Verification items for the finished model (mm, model axes). A direction names the side the tool comes from. Give positions to 0.01 mm unless a question says otherwise; leave off trailing zeros. Loops run counter-clockwise (first coordinate to the right, second up) from the corner with the lowest first, then second, coordinate; pieces in that order, holes last. Notation, with made-up numbers: (56, 85) -> (112, 85) arc R6 ccw to (112, 95) -> close; hole circle Ø11 at (82.25, -28.5). An arc over 180 degrees is marked (long way). Answer in a Markdown table with one row per item. Add a question column.
Q1. Set-up check for faces 1 (the face through (-66.1, 6, 12.7)), 2 (the face through (71, 0, 12.7)), 3 (the face through (0, 0, 25.4)): record each of +Z, -Z, +X, -X, +Y, -Y from which the full face is reachable in a straight line by a thin tool's end or side.
Q2. Section check D-D on y = 23. Enter the section's corners in (x, z).
Q3. Section check B-B on z = 10.5. Enter the section's corners in (x, y).
Q4. Gauge pin test, flat ends, axial feed: P1, Ø4, axis at x = -51.5, z = 6, coming from the -Y side; P2, Ø4, axis at x = 56.5, z = 5.5, coming from the +Y side; P3, Ø23, axis at x = 72, y = -5.5, coming from the +Z side. Record the tip position at first contact, or that the pin passes through.
Q5. Material ranges on probe 1 along Y at (x, z) = (63, 8); probe 2 along Z at (x, y) = (-52, -19); probe 3 along X at (y, z) = (29, 12), recorded low to high.
Q6. Section check C-C on x = 0. Enter the section's corners in (y, z).
Q7. Section check A-A on y = 0. Enter the section's corners in (x, z), and give its area (3 significant figures).
Autodesk Fusion 360 part; units mm, degrees
sketch "Sketch1" plane through (0, 0, 0) normal (0, 0, 1) x (1, 0, 0) in component "u-Bracket"
  line L0 (-63.5, -25.4) -> (63.5, -25.4)
  arc A0 (63.5, -25.4) -> (63.5, 25.4) centre (63.5, 0) ccw
  line L1 (63.5, 25.4) -> (-63.5, 25.4)
  arc A1 (-63.5, 25.4) -> (-63.5, -25.4) centre (-63.5, 0) ccw
  line L2 (-63.5, 0) -> (63.5, 0) construction
  circle A2 centre (63.5, 0) radius 6.35
  circle A3 centre (-63.5, 0) radius 6.35
  dimension "d1" = 127
  dimension "d2" = 12.7
  dimension "d3" = 12.7
  dimension "d4" = 25.4
  dimension "d5" = 63.5
extrude "Extrude2" add sketch "Sketch1" along normal blind 12.7 makes body 1 in component "u-Bracket"
extrude "Extrude1" add sketch "Sketch1" along normal blind 12.7 separate body makes body 2 in component "u-Bracket"
sketch "Sketch2" plane through (0, 0, 0) normal (0, 1, 0) x (1, 0, 0) in component "u-Bracket"
  circle A0 centre (0, 0) radius 44.45
  line L0 (-44.45, 0) -> (44.45, 0)
  dimension "d10" = 88.9
extrude "Extrude3" add sketch "Sketch2" along normal mid plane 63.5 contours A0 L0 picked at (-7.4083, -12.8316) bodies 1 2 in component "u-Bracket"
sketch "Sketch3" plane through (0, -31.75, 0) normal (0, -1, 0) x (1, 0, 0) in component "u-Bracket"
  arc A0 (44.45, 0) -> (-44.45, 0) centre (0, 0) ccw
  line L0 (-44.45, 0) -> (44.45, 0)
  line L1 (-25.4, 0) -> (25.4, 0)
  line L2 (25.4, 0) -> (25.4, 25.4)
  line L3 (25.4, 25.4) -> (-25.4, 25.4)
  line L4 (-25.4, 25.4) -> (-25.4, 0)
  line L5 (-63.5, 0) -> (63.5, 0)
  dimension "d13" = 50.8
  dimension "d14" = 25.4
extrude "Extrude4" cut sketch "Sketch3" against normal through all contours L0 L1 L2 L3 L4 L5 bodies 1 in component "u-Bracket"
sketch "Sketch4" plane through (0, 0, 25.4) normal (0, 0, -1) x (1, 0, 0) in component "u-Bracket"
  line L0 (-25.4, -31.75) -> (25.4, -31.75)
  line L1 (25.4, -31.75) -> (25.4, 31.75)
  line L2 (25.4, 31.75) -> (-25.4, 31.75)
  line L3 (-25.4, 31.75) -> (-25.4, -31.75)
  circle A0 centre (0, 0) radius 3.175
  dimension "d16" = 6.35
extrude "Extrude5" cut sketch "Sketch4" along normal through all contours A0 bodies 1 in component "u-Bracket"
component "u-Bracket" placed x (1, 0, 0) y (0, 1, 0) z (0, 0, 1) at (0, 0, 0)
equation "d5 = d1 / 2"
Taken from the geometry:
| question | item | result |
|---|---|---|
| 1 | face 1 | +Z, -X, +Y, -Y |
| 1 | face 2 | +Z, +X, +Y, -Y |
| 1 | face 3 | -Z, +Y, -Y |
| 2 | outline | (-74.28, 0) -> (-25.4, 0) -> (-25.4, 25.4) -> (25.4, 25.4) -> (25.4, 0) -> (74.28, 0) -> (74.28, 12.7) -> (42.6, 12.7) arc R44.45 ccw to (-42.6, 12.7) -> (-74.28, 12.7) -> close |
| 3 | outline | (-63.5, -25.4) -> (-43.19, -25.4) -> (-43.19, -31.75) -> (-25.4, -31.75) -> (-25.4, 31.75) -> (-43.19, 31.75) -> (-43.19, 25.4) -> (-63.5, 25.4) arc R25.4 ccw to start; (25.4, -31.75) -> (43.19, -31.75) -> (43.19, -25.4) -> (63.5, -25.4) arc R25.4 ccw to (63.5, 25.4) -> (43.19, 25.4) -> (43.19, 31.75) -> (25.4, 31.75) -> close; hole circle Ø12.7 at (-63.5, 0); hole circle Ø12.7 at (63.5, 0) |
| 4 | P1 | stops at y = -25.4 |
| 4 | P2 | stops at y = 25.4 |
| 4 | P3 | stops at z = 12.7 |
| 5 | probe 1 | y = -25.4 to -6.33, 6.33 to 25.4 |
| 5 | probe 2 | z = 0 to 12.7 |
| 5 | probe 3 | x = -42.8 to -25.4, 25.4 to 42.8 |
| 6 | outline | (-31.75, 25.4) -> (31.75, 25.4) -> (31.75, 44.45) -> (-31.75, 44.45) -> close |
| 7 | outline | (-88.9, 0) -> (-69.85, 0) -> (-69.85, 12.7) -> (-88.9, 12.7) -> close; (-57.15, 0) -> (-25.4, 0) -> (-25.4, 25.4) -> (25.4, 25.4) -> (25.4, 0) -> (57.15, 0) -> (57.15, 12.7) -> (42.6, 12.7) arc R44.45 ccw to (-42.6, 12.7) -> (-57.15, 12.7) -> close; (69.85, 0) -> (88.9, 0) -> (88.9, 12.7) -> (69.85, 12.7) -> close |
| 7 | area | 2,640 mm² |
